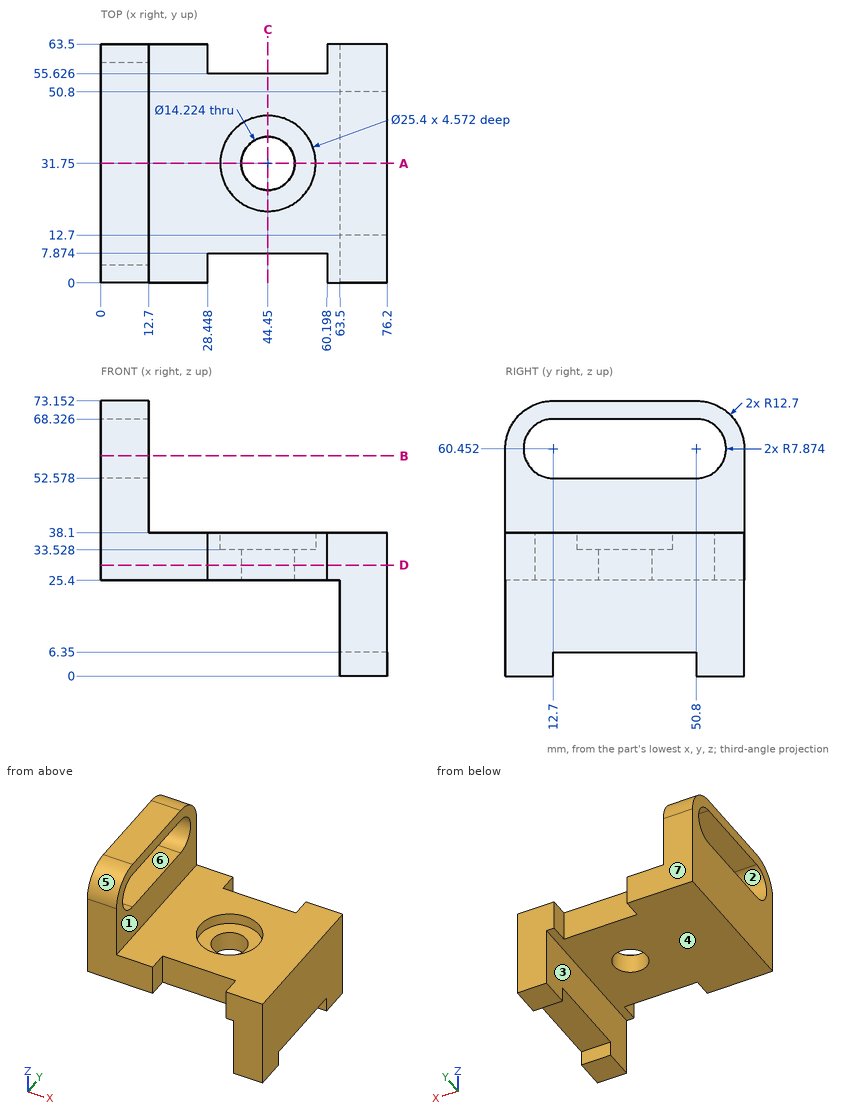
Verification items for this drawing (mm, ordinates from the low corner). A direction names the side the tool comes from. Give positions to 0.01 mm unless a question says otherwise; leave off trailing zeros. Write each loop counter-clockwise with the first axis right and the second up, starting at its lowest first coordinate (ties: lowest second). Pieces come first, ordered by that corner, then holes.
1) Section check A-A, the plane y = 31.75. Record the boundary of the cut face in (x, z), and give its area (3 significant figures).
2) Section check C-C, the plane x = 44.45. Record the boundary of the cut face in (y, z), and give its area (3 significant figures).
3) Release check for a two-part mould opening along Z. For the marked faces 4, 5, 6 and 7 record: pulls with the +Z half, pulls with the -Z half, needs draft (parallel to the pull), parting line crosses it, or undercut.
4) Gauge pin test, flat ends, axial feed: pin 1 (4 mm diameter, centred on x = 63.5, z = 17.5, fed in from -Y); pin 2 (1 mm diameter, centred on x = 31, y = 12.5, fed in from +Z); pin 3 (10 mm diameter, centred on x = 62.5, y = 32, fed in from -Z); pin 4 (4 mm diameter, centred on x = 44.5, z = 31, fed in from -Y). Record the tip position at first contact, or that the pin passes through.
5) Section check D-D, the plane z = 29.5. Record the boundary of the cut face in (x, y).
6) Material ranges on L1, parallel to Y at x = 44, z = 35; L2, parallel to Y at x = 44.45, z = 31.25; L3, parallel to X at y = 31.75, z = 30.75, recorded low to high.
7) Section check B-B, the plane z = 58.5. Record the boundary of the cut face in (x, y).
8) Access from +Z, -Z, +X, -X, +Y, -Y to the whole of each face (thin tool, end or side, straight path). Record for the marked faces 1, 2 and 3.
Computed:
1. outline: (0, 25.4) - (37.34, 25.4) - (37.34, 33.53) - (31.75, 33.53) - (31.75, 38.1) - (12.7, 38.1) - (12.7, 52.58) - (0, 52.58) - close; (0, 68.33) - (12.7, 68.33) - (12.7, 73.15) - (0, 73.15) - close; (51.56, 25.4) - (63.5, 25.4) - (63.5, 6.35) - (76.2, 6.35) - (76.2, 38.1) - (57.15, 38.1) - (57.15, 33.53) - (51.56, 33.53) - close
1. area: 1,220 mm2
2. outline: (7.87, 25.4) - (24.64, 25.4) - (24.64, 33.53) - (19.05, 33.53) - (19.05, 38.1) - (7.87, 38.1) - close; (38.86, 25.4) - (55.63, 25.4) - (55.63, 38.1) - (44.45, 38.1) - (44.45, 33.53) - (38.86, 33.53) - close
2. area: 375 mm2
3. face 4: pulls with the -Z half
3. face 5: pulls with the +Z half
3. face 6: undercut
3. face 7: needs draft
4. pin 1: stops at y = 0
4. pin 2: stops at z = 38.1
4. pin 3: stops at z = 6.35
4. pin 4: stops at y = 7.87
5. outline: (0, 0) - (28.45, 0) - (28.45, 7.87) - (60.2, 7.87) - (60.2, 0) - (76.2, 0) - (76.2, 63.5) - (60.2, 63.5) - (60.2, 55.63) - (28.45, 55.63) - (28.45, 63.5) - (0, 63.5) - close; hole circle Ø14.22 at (44.45, 31.75)
6. L1: y = 7.87 to 19.06, 44.44 to 55.63
6. L2: y = 7.87 to 24.64, 38.86 to 55.63
6. L3: x = 0 to 37.34, 51.56 to 76.2
7. outline: (0, 0) - (12.7, 0) - (12.7, 5.07) - (0, 5.07) - close; (0, 58.43) - (12.7, 58.43) - (12.7, 63.5) - (0, 63.5) - close
8. face 1: +Z, +X, +Y, -Y
8. face 2: +X, -X
8. face 3: -Z, -X, +Y, -Y
